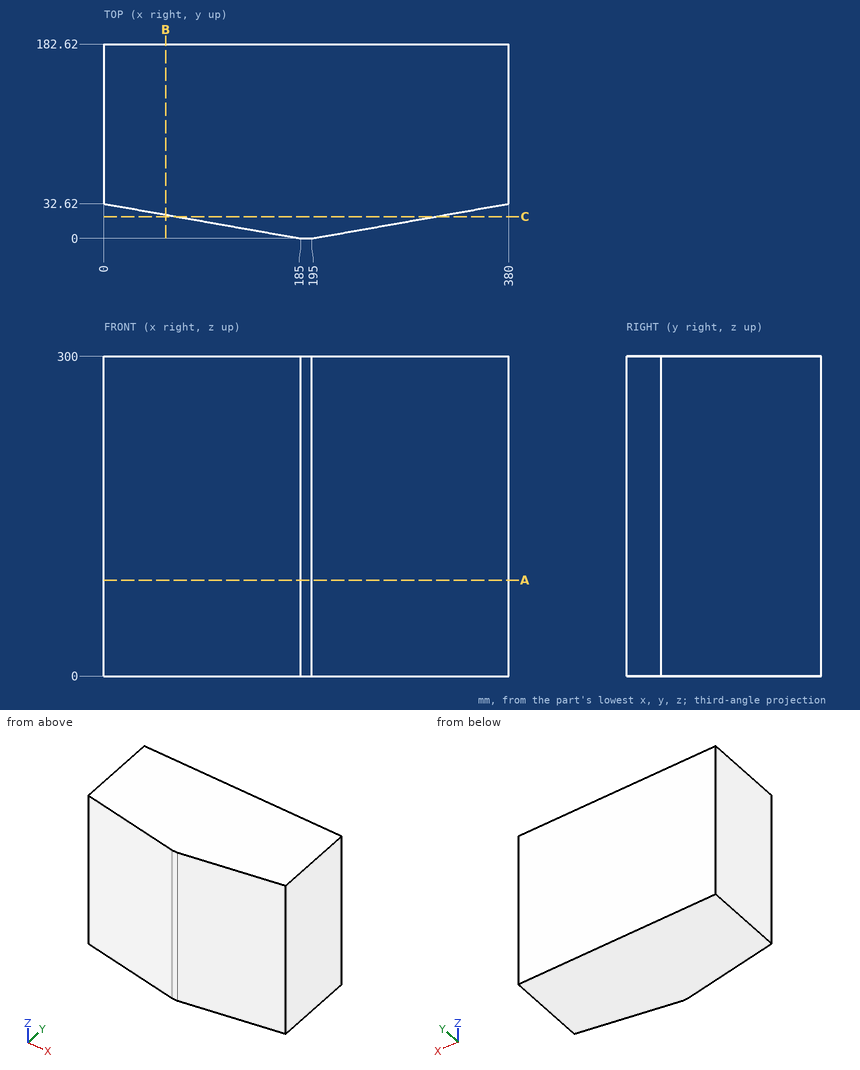
Geometry: see drawing. Coordinates: mm, zero at the bounding-box minimum. Round coordinates to 2 decimals unless told otherwise and drop trailing zeros. Loops run counter-clockwise (first coordinate to the right, second up) from the corner with the lowest first, then second, coordinate; pieces in that order, holes last.
(1) Contact query for flat-ended pins moving along their axis: pin 1 Ø10 at (x, z) = (136.5, 44.5) entering from -Y; pin 2 Ø10 at (x, z) = (284, 171) entering from -Y. Output: stop coordinate, or through.
From the geometry:
pin 1: stops at y = 7.67
pin 2: stops at y = 14.81
(2) Section query A-A (z = 90). Output: boundary loops of the cut face in (x, y), and give its area (3 significant figures).
From the geometry:
outline: (0, 32.62) - (185, 0) - (195, 0) - (380, 32.62) - (380, 182.62) - (0, 182.62) - close
area: 63,400 mm2
(3) Section query B-B (x = 58). Output: boundary loops of the cut face in (y, z), and give its area (3 significant figures).
From the geometry:
outline: (22.39, 0) - (182.62, 0) - (182.62, 300) - (22.39, 300) - close
area: 48,100 mm2
(4) Section query C-C (y = 20.5). Output: boundary loops of the cut face in (x, z), and give its area (3 significant figures).
From the geometry:
outline: (68.74, 0) - (311.26, 0) - (311.26, 300) - (68.74, 300) - close
area: 72,800 mm2
(5) Material intervals for probe 1 along Y at (x, z) = (199.5, 205.5); probe 2 along Y at (x, z) = (49, 246.5), sorted ascending.
From the geometry:
probe 1: y = 0.79 to 182.62
probe 2: y = 23.98 to 182.62
